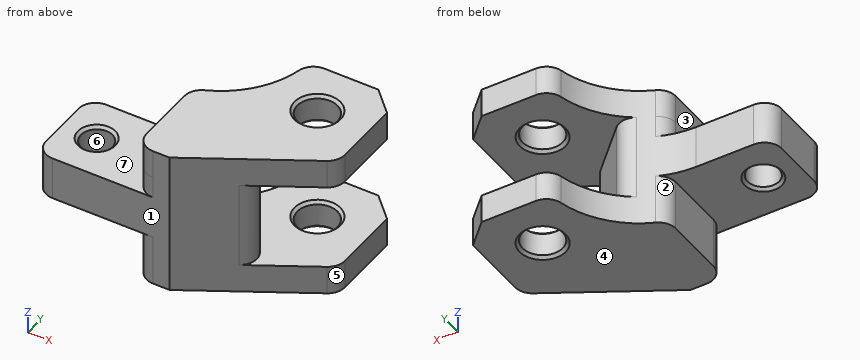
```python
from build123d import *

# Parameters (mm, degrees)
BOSS_EXTRUDE1_DEPTH       = 10
FILLET1_R                 = 6
FILLET2_R                 = 6
FILLET3_R                 = 6
CUT_EXTRUDE1_REACH        = 92.604
SKETCH4_R                 = 7.000000000000001
CHAMFER1_SIZE             = 1
CHAMFER2_SIZE             = 1
BOSS_EXTRUDE2_DEPTH       = 7.5
FILLET4_R                 = 6
SKETCH5_R                 = 5.5
CUT_EXTRUDE2_DEPTH        = 15
CHAMFER3_SIZE             = 1
BOSS_EXTRUDE3_DEPTH       = 15
FILLET5_R                 = 6
FILLET1_OF_MIRROR16_R     = 6
FILLET2_OF_MIRROR16_R     = 6
FILLET3_OF_MIRROR16_R     = 6
CHAMFER1_OF_MIRROR16_SIZE = 1
CHAMFER2_OF_MIRROR16_SIZE = 1


with BuildPart() as part:
    # Sketch3 → Boss-Extrude1 (new body)
    with BuildSketch(Plane.XY.offset(15)):
        with BuildLine():
            Line((45.93743884534262, 45.00000000000001), (69.99999999999996, 45))
            Line((69.99999999999996, 45), (77.99999999999999, 37))
            Line((77.99999999999999, 37), (77.99999999999999, 9.999999999999998))
            Line((77.99999999999999, 9.999999999999998), (34.69872981077818, -15.000000000000004))
            Line((34.69872981077818, -15.000000000000004), (22.999999999999996, -15.000000000000005))
            Line((22.999999999999996, -15.000000000000005), (22.99999999999999, 16.291694934431824))
            ThreePointArc((22.99999999999999, 16.291694934431824), (39.00020339394204, 27.025270208047246), (45.93743884534262, 45.00000000000001))
        make_face()
    boss_extrude1 = extrude(amount=BOSS_EXTRUDE1_DEPTH)

    # Fillet1
    fillet1_edges = [part.edges().sort_by_distance(p)[0] for p in [
        (45.93743884534262, 45.00000000000001, 20),
    ]]
    fillet(fillet1_edges, radius=FILLET1_R)

    # Fillet2
    fillet2_edges = [part.edges().sort_by_distance(p)[0] for p in [
        (22.999999999999996, -15.000000000000005, 20),
    ]]
    fillet(fillet2_edges, radius=FILLET2_R)

    # Fillet3
    fillet3_edges = [part.edges().sort_by_distance(p)[0] for p in [
        (77.99999999999999, 9.999999999999998, 20),
        (22.999999999999993, 16.29169493443182, 20),
    ]]
    fillet(fillet3_edges, radius=FILLET3_R)

    # Sketch4 → Cut-Extrude1 (cut, up to next)
    with BuildSketch(Plane.XY.offset(25), mode=Mode.PRIVATE) as cut_extrude1_sk1:
        with Locations((59.999999999999986, 27)):
            Circle(SKETCH4_R)
    cut_extrude1_tool1 = extrude(cut_extrude1_sk1.sketch, amount=-CUT_EXTRUDE1_REACH, mode=Mode.PRIVATE) & part.part
    cut_extrude1 = cut_extrude1_tool1.solids().sort_by_distance((60, 27, 25))[0]
    add(cut_extrude1, mode=Mode.SUBTRACT)

    # Chamfer1
    chamfer1_edges = [part.edges().sort_by_distance(p)[0] for p in [
        (52.999999999999986, 27, 25),
    ]]
    chamfer(chamfer1_edges, length=CHAMFER1_SIZE)

    # Chamfer2
    chamfer2_edges = [part.edges().sort_by_distance(p)[0] for p in [
        (52.999999999999986, 27, 15),
    ]]
    chamfer(chamfer2_edges, length=CHAMFER2_SIZE)



with BuildPart() as body_2:
    # Sketch2 → Boss-Extrude2 (new, symmetric)
    with BuildSketch(Plane.XY):
        with BuildLine():
            Line((-12.000000000000009, 14.999999999999996), (13.999999999999993, 15.000000000000002))
            ThreePointArc((13.999999999999993, 15.000000000000002), (23.496761564827036, 16.441670206295278), (32.13782324188529, 20.636780013698527))
            Line((32.13782324188529, 20.636780013698527), (55.66799332242584, -2.893390066842031))
            Line((55.66799332242584, -2.893390066842031), (34.69872981077818, -15.000000000000004))
            Line((34.69872981077818, -15.000000000000004), (-12, -15.000000000000004))
            Line((-12, -15.000000000000004), (-12.000000000000009, 14.999999999999996))
        make_face()
    extrude(amount=BOSS_EXTRUDE2_DEPTH, both=True)

    # Fillet4
    fillet4_edges = [body_2.edges().sort_by_distance(p)[0] for p in [
        (-12.000000000000009, 14.999999999999996, 0),
        (32.13782324188529, 20.636780013698527, 0),
        (55.66799332242584, -2.893390066842031, 0),
        (-12, -15.000000000000004, 0),
    ]]
    fillet(fillet4_edges, radius=FILLET4_R)

    # Sketch5 → Cut-Extrude2 (cut)
    with BuildSketch(Plane.XY.offset(7.5)):
        Circle(SKETCH5_R)
    extrude(amount=-CUT_EXTRUDE2_DEPTH, mode=Mode.SUBTRACT)

    # Chamfer3
    chamfer3_edges = [body_2.edges().sort_by_distance(p)[0] for p in [
        (-5.5, 3.12e-15, 7.5),
        (-5.5, 3.12e-15, -7.5),
    ]]
    chamfer(chamfer3_edges, length=CHAMFER3_SIZE)


with BuildPart() as part_1:
    add(part.part)

    add(body_2.part)  # Boss-Extrude3 merges body 2
    # Sketch6 → Boss-Extrude3 (add, symmetric)
    with BuildSketch(Plane.XY):
        with BuildLine():
            Line((22.99999999999999, -15.000000000000004), (22.999999999999996, 16.291694934431828))
            ThreePointArc((22.999999999999996, 16.291694934431828), (29.533716734106008, 19.023158784012917), (35.30667046294364, 23.124787042132485))
            Line((35.30667046294364, 23.124787042132485), (59.25429521109807, -0.8228377060218555))
            Line((59.25429521109807, -0.8228377060218555), (34.69872981077818, -15.000000000000004))
            Line((34.69872981077818, -15.000000000000004), (22.99999999999999, -15.000000000000004))
        make_face()
    extrude(amount=BOSS_EXTRUDE3_DEPTH, both=True)

    # Fillet5
    fillet5_edges = [part_1.edges().sort_by_distance(p)[0] for p in [
        (22.99999999999999, -15.000000000000004, -11.25),
        (22.99999999999999, -15.000000000000004, 11.25),
        (22.999999999999996, 16.291694934431828, -11.25),
        (22.999999999999996, 16.291694934431828, 11.25),
        (59.25429521109807, -0.8228377060218555, 0),
        (35.30667046294364, 23.12478704213249, 0),
    ]]
    fillet(fillet5_edges, radius=FILLET5_R)


with BuildPart() as mirror16_1:
    # Mirror16: Boss-Extrude1 across plane
    add(boss_extrude1.mirror(Plane.XY))

    # Mirror16 2: Cut-Extrude1 across plane
    add(cut_extrude1.mirror(Plane.XY), mode=Mode.SUBTRACT)

    # Fillet1 of Mirror16
    fillet1_of_mirror16_edges = [mirror16_1.edges().sort_by_distance(p)[0] for p in [
        (45.93743884534262, 45.00000000000001, -20),
    ]]
    fillet(fillet1_of_mirror16_edges, radius=FILLET1_OF_MIRROR16_R)

    # Fillet2 of Mirror16
    fillet2_of_mirror16_edges = [mirror16_1.edges().sort_by_distance(p)[0] for p in [
        (22.999999999999996, -15.000000000000005, -20),
    ]]
    fillet(fillet2_of_mirror16_edges, radius=FILLET2_OF_MIRROR16_R)

    # Fillet3 of Mirror16
    fillet3_of_mirror16_edges = [mirror16_1.edges().sort_by_distance(p)[0] for p in [
        (77.99999999999999, 9.999999999999998, -20),
        (22.999999999999993, 16.29169493443182, -20),
    ]]
    fillet(fillet3_of_mirror16_edges, radius=FILLET3_OF_MIRROR16_R)

    # Chamfer1 of Mirror16
    chamfer1_of_mirror16_edges = [mirror16_1.edges().sort_by_distance(p)[0] for p in [
        (52.999999999999986, 27, -25),
    ]]
    chamfer(chamfer1_of_mirror16_edges, length=CHAMFER1_OF_MIRROR16_SIZE)

    # Chamfer2 of Mirror16
    chamfer2_of_mirror16_edges = [mirror16_1.edges().sort_by_distance(p)[0] for p in [
        (52.999999999999986, 27, -15),
    ]]
    chamfer(chamfer2_of_mirror16_edges, length=CHAMFER2_OF_MIRROR16_SIZE)


with BuildPart() as part_2:
    add(part_1.part)

    # Mirror16 united with what the copies tou: union Mirror16_1
    add(mirror16_1.part)


solid = part_2.part
```
The listing builds one solid part. Answer for the finished solid, in the listing's coordinates (mm). Face numbers are marked on the shaded views. A direction names the side the tool comes from. Coordinates: 2 decimals unless noted, no trailing zeros. Write each loop counter-clockwise with the first axis right and the second up, starting at its lowest first coordinate (ties: lowest second). Pieces come first, ordered by that corner, then holes. Notation, with made-up numbers: (74, 52) - (125, 52) arc R18 ccw to (125, 73) - close; hole circle Ø6 at (-14, -39). An arc over 180 degrees is marked (long way). Return JSON: item names as keys, results as strings. Group by question number.
Q1. Flat-ended cylindrical pins translate along their axes: pin 1 Ø8 at (y, z) = (9.5, 5.5) entering from +X; pin 2 Ø2 at (x, y) = (9.5, 14) entering from +Z; pin 3 Ø12 at (x, z) = (19.5, -4.5) entering from +Y. Find the tip coordinate at first contact, or state that the pin passes through.
Q2. Find the intervals of material crossed by line 1 along Y through (x, z) = (0, -1); line 2 along Z through (x, y) = (-1, -7.5); line 3 along Y through (x, z) = (11, 5.5), in increasing order. Write a range as [from, to].
Q3. For a pull along X with two mould halves and no side action, classify the marked faces 5, 6 and 7 as +X half, -X half, draft (parallel to the pull), parting line (faces both ways), or undercut.
Q4. The part is cut by section D-D on y = 0. Write down the section's boundary in (x, z).
Q5. The part is cut by section C-C on y = 27. Write down the section's boundary in (x, z), and give its area (3 significant figures).
Q6. The part is cut by section A-A on x = 0. Write down the section's boundary in (y, z).
Q7. Which of the six approach directions +Z, -Z, +X, -X, +Y, -Y give full straight-line access (tool end or side, diameter ignored) to the marked faces 1, 2, 3 and 4?
Q8. The part is cut by section B-B on z = -17. Write down the section's boundary in (x, y).
Evaluation:
{
 "1": {"pin 1": "stops at x = 52.93", "pin 2": "stops at z = 7.5", "pin 3": "stops at y = 17.14"},
 "2": {"line 1": "y = [-15, -5.5], [5.5, 15]", "line 2": "z = [-7.5, 7.5]", "line 3": "y = [-15, 15]"},
 "3": {"face 5": "+X half", "face 6": "undercut", "face 7": "draft"},
 "4": {"outline": "(-12, -7.5) - (-6.5, -7.5) - (-5.5, -6.5) - (-5.5, 6.5) - (-6.5, 7.5) - (-12, 7.5) - close; (5.5, -6.5) - (6.5, -7.5) - (23, -7.5) - (23, -25) - (60.68, -25) - (60.68, -15) - (55.46, -15) - (55.46, 15) - (60.68, 15) - (60.68, 25) - (23, 25) - (23, 7.5) - (6.5, 7.5) - (5.5, 6.5) - close"},
 "5": {"outline": "(38.98, -25) - (52, -25) - (53, -24) - (53, -16) - (52, -15) - (38.98, -15) - close; (38.98, 15) - (52, 15) - (53, 16) - (53, 24) - (52, 25) - (38.98, 25) - close; (67, -24) - (68, -25) - (78, -25) - (78, -15) - (68, -15) - (67, -16) - close; (67, 16) - (68, 15) - (78, 15) - (78, 25) - (68, 25) - (67, 24) - close", "area": "496 mm2"},
 "6": {"outline": "(-15, -7.5) - (-6.5, -7.5) - (-5.5, -6.5) - (-5.5, 6.5) - (-6.5, 7.5) - (-15, 7.5) - close; (5.5, -6.5) - (6.5, -7.5) - (15, -7.5) - (15, 7.5) - (6.5, 7.5) - (5.5, 6.5) - close"},
 "7": {"face 1": "+Z, -Z, +X, -X, -Y", "face 2": "-Z, -X, +Y", "face 3": "+Z, -X, +Y, -Y", "face 4": "-Z, +X, -X, +Y, -Y"},
 "8": {"outline": "(23, -9) arc R6 ccw to (29, -15) - (34.7, -15) - (75, 8.27) arc R6 ccw to (78, 13.46) - (78, 37) - (70, 45) - (51.15, 45) arc R6 ccw to (45.28, 40.26) arc R32 cw to (26.63, 17.6) arc R6 ccw to (23, 12.09) - close; hole circle Ø14 at (60, 27)"}
}
